from build123d import *

# Parameters (mm, degrees)
BOSS_EXTRUDE1_DEPTH      = 0.762
BOSS_EXTRUDE1_DEPTH_BACK = 0.762
SKETCH4_R                = 2.3495
CUT_EXTRUDE1_DEPTH       = 1.762
CUT_EXTRUDE1_DEPTH_BACK  = 1.762
SKETCH5_R                = 3.5433
CUT_EXTRUDE2_DEPTH       = 2.524
CUT_EXTRUDE2_TAPER       = 41


with BuildPart() as part:
    # Sketch3 → Boss-Extrude1 (new body, two sides)
    with BuildSketch(Plane.XY) as boss_extrude1_sk:
        Polygon((-31.75, 31.75), (-19.05, 31.75), (-19.05, -19.05), (31.75, -19.05), (31.75, -31.75), (-31.75, -31.75), align=None)
    extrude(amount=BOSS_EXTRUDE1_DEPTH)
    extrude(boss_extrude1_sk.sketch, amount=-BOSS_EXTRUDE1_DEPTH_BACK)

    # Sketch4 → Cut-Extrude1 (cut, two sides)
    with BuildSketch(Plane.XY) as cut_extrude1_sk:
        with Locations((-25.4, 19.05)):
            Circle(SKETCH4_R)
        with Locations((-25.4, -9.652)):
            Circle(SKETCH4_R)
        with Locations((-9.652, -25.4)):
            Circle(SKETCH4_R)
        with Locations((19.05, -25.4)):
            Circle(SKETCH4_R)
    extrude(amount=CUT_EXTRUDE1_DEPTH, mode=Mode.SUBTRACT)
    extrude(cut_extrude1_sk.sketch, amount=-CUT_EXTRUDE1_DEPTH_BACK, mode=Mode.SUBTRACT)

    # Sketch5 → Cut-Extrude2 (cut, through all)
    with BuildSketch(Plane.XY.offset(0.762)):
        with Locations((-25.4, 19.05)):
            Circle(SKETCH5_R)
        with Locations((-25.4, -9.652)):
            Circle(SKETCH5_R)
        with Locations((-9.652, -25.4)):
            Circle(SKETCH5_R)
        with Locations((19.05, -25.4)):
            Circle(SKETCH5_R)
    extrude(amount=-CUT_EXTRUDE2_DEPTH, taper=CUT_EXTRUDE2_TAPER, mode=Mode.SUBTRACT)


solid = part.part
The listing builds one solid part. Answer for the finished solid, in the listing's coordinates (mm). A direction names the side the tool comes from. Give positions to 0.01 mm unless a question says otherwise; leave off trailing zeros. Loops run counter-clockwise (first coordinate to the right, second up) from the corner with the lowest first, then second, coordinate; pieces in that order, holes last. Notation, with made-up numbers: M 46.25,-19 L 88.25,-19 A24 cw 88.25,5 Z; hole C -26.5,10 d9. An arc over 180 degrees is marked long. Answer as CSV lines item,"result".
Item 1: The part is cut by section A-A (x = -25.4). Give the vertices of the cut face in (y, z), and give its area (3 significant figures).
Values follow:
outline,"M -31.75,-0.76 L -12,-0.76 L -12,-0.61 L -13.2,0.76 L -31.75,0.76 Z; M -7.3,-0.76 L 16.7,-0.76 L 16.7,-0.61 L 15.51,0.76 L -6.11,0.76 L -7.3,-0.61 Z; M 21.4,-0.76 L 31.75,-0.76 L 31.75,0.76 L 22.59,0.76 L 21.4,-0.61 Z"
area,"79.2 mm^2"
Item 2: The part is cut by section D-D (y = 2.5). Give the vertices of the cut face in (x, z).
Values follow:
outline,"M -31.75,-0.76 L -19.05,-0.76 L -19.05,0.76 L -31.75,0.76 Z"
Item 3: The part is cut by section C-C (z = -0.05). Give the vertices of the cut face in (x, y).
Values follow:
outline,"M -31.75,-31.75 L 31.75,-31.75 L 31.75,-19.05 L -19.05,-19.05 L -19.05,31.75 L -31.75,31.75 Z; hole C -25.4,-9.65 d5.67; hole C -25.4,19.05 d5.67; hole C -9.65,-25.4 d5.67; hole C 19.05,-25.4 d5.67"
Item 4: The part is cut by section B-B (x = 19.05). Give the vertices of the cut face in (y, z).
Values follow:
outline,"M -31.75,-0.76 L -27.75,-0.76 L -27.75,-0.61 L -28.94,0.76 L -31.75,0.76 Z; M -23.05,-0.76 L -19.05,-0.76 L -19.05,0.76 L -21.86,0.76 L -23.05,-0.61 Z"
Item 5: Straight lines are drawn through the part: line 1 along Y through (x, z) = (-25.4, -0.6); line 2 along Y through (x, z) = (-23.5, 0.7); line 3 along Y through (x, z) = (19.05, -0.65). For each, find the intervals that lie inside material, in ascending order. Write a range as [from, to].
Values follow:
line 1,"y = [-31.75, -12.01], [-7.29, 16.69], [21.41, 31.75]"
line 2,"y = [-31.75, -12.58], [-6.73, 16.12], [21.98, 31.75]"
line 3,"y = [-31.75, -27.75], [-23.05, -19.05]"
Item 6: Which of the six approach directions +Z, -Z, +X, -X, +Y, -Y give full straight-line access (tool end or side, diameter ignored) to faces 1 (the flat face through (6, -19.05, 0)), 2 (the flat face through (31.75, -25, 0))?
Values follow:
face 1,"+Z, -Z, +X, +Y"
face 2,"+Z, -Z, +X, +Y, -Y"
Item 7: Given pin 1 Ø6 at (x, y) = (-9.652, -25.4) entering from -Z; pin 2 Ø4 at (x, y) = (-25.4, 19.05) entering from -Z; pin 3 Ø0.5 at (y, z) = (-0.5, 0) entering from +X; pin 4 Ø0.5 at (x, z) = (-4.5, 0.5) entering from +Y, each flat-ended and moving along its own axis, determine where each tip first touches the part or whether it passes through.
Values follow:
pin 1,"stops at z = -0.76"
pin 2,"passes through"
pin 3,"stops at x = -19.05"
pin 4,"stops at y = -19.05"
